```python
from build123d import *

# Parameters (mm, degrees)
BOSS_EXTRUDE1_DEPTH = 4
CUT_EXTRUDE1_REACH  = 42.756
SKETCH2_R           = 2
SKETCH2_R_2         = 2.75
SKETCH2_R_3         = 15
SKETCH4_W           = 4
SKETCH4_H           = 51.1
BOSS_EXTRUDE2_DEPTH = 37
CUT_EXTRUDE2_REACH  = 75.219
SKETCH5_R           = 2.75
CHAMFER2_SIZE       = 30


with BuildPart() as part:
    # Sketch1 → Boss-Extrude1 (new body)
    with BuildSketch(Plane.XY):
        Polygon((-31.5, 21.15), (-31.5, -21.15), (-31.5, -25.55), (31.5, -25.55), (31.5, -21.15), (31.5, 21.15), (31.5, 25.55), (-31.5, 25.55), align=None)
    extrude(amount=BOSS_EXTRUDE1_DEPTH)

    # Sketch2 → Cut-Extrude1 (cut, up to next)
    with BuildSketch(Plane.XY.offset(4), mode=Mode.PRIVATE) as cut_extrude1_sk1:
        with Locations((-5.2, 15.55)):
            Circle(SKETCH2_R)
    cut_extrude1_tool1 = extrude(cut_extrude1_sk1.sketch, amount=-CUT_EXTRUDE1_REACH, mode=Mode.PRIVATE) & part.part
    # Sketch2 → Cut-Extrude1 (cut, up to next)
    with BuildSketch(Plane.XY.offset(4), mode=Mode.PRIVATE) as cut_extrude1_sk2:
        with Locations((25.9, 15.55)):
            Circle(SKETCH2_R)
    cut_extrude1_tool2 = extrude(cut_extrude1_sk2.sketch, amount=-CUT_EXTRUDE1_REACH, mode=Mode.PRIVATE) & part.part
    # Sketch2 → Cut-Extrude1 (cut, up to next)
    with BuildSketch(Plane.XY.offset(4), mode=Mode.PRIVATE) as cut_extrude1_sk3:
        with Locations((25.9, -15.55)):
            Circle(SKETCH2_R)
    cut_extrude1_tool3 = extrude(cut_extrude1_sk3.sketch, amount=-CUT_EXTRUDE1_REACH, mode=Mode.PRIVATE) & part.part
    # Sketch2 → Cut-Extrude1 (cut, up to next)
    with BuildSketch(Plane.XY.offset(4), mode=Mode.PRIVATE) as cut_extrude1_sk4:
        with Locations((-5.2, -15.55)):
            Circle(SKETCH2_R)
    cut_extrude1_tool4 = extrude(cut_extrude1_sk4.sketch, amount=-CUT_EXTRUDE1_REACH, mode=Mode.PRIVATE) & part.part
    # Sketch2 → Cut-Extrude1 (cut, up to next)
    with BuildSketch(Plane.XY.offset(4), mode=Mode.PRIVATE) as cut_extrude1_sk5:
        with Locations((-21.5, 15.55)):
            Circle(SKETCH2_R_2)
    cut_extrude1_tool5 = extrude(cut_extrude1_sk5.sketch, amount=-CUT_EXTRUDE1_REACH, mode=Mode.PRIVATE) & part.part
    # Sketch2 → Cut-Extrude1 (cut, up to next)
    with BuildSketch(Plane.XY.offset(4), mode=Mode.PRIVATE) as cut_extrude1_sk6:
        with Locations((-21.5, -15.55)):
            Circle(SKETCH2_R_2)
    cut_extrude1_tool6 = extrude(cut_extrude1_sk6.sketch, amount=-CUT_EXTRUDE1_REACH, mode=Mode.PRIVATE) & part.part
    # Sketch2 → Cut-Extrude1 (cut, up to next)
    with BuildSketch(Plane.XY.offset(4), mode=Mode.PRIVATE) as cut_extrude1_sk7:
        with Locations((10.35, 0)):
            Circle(SKETCH2_R_3)
    cut_extrude1_tool7 = extrude(cut_extrude1_sk7.sketch, amount=-CUT_EXTRUDE1_REACH, mode=Mode.PRIVATE) & part.part
    add(cut_extrude1_tool1.solids().sort_by_distance((-5.2, 15.55, 4))[0], mode=Mode.SUBTRACT)
    add(cut_extrude1_tool2.solids().sort_by_distance((25.9, 15.55, 4))[0], mode=Mode.SUBTRACT)
    add(cut_extrude1_tool3.solids().sort_by_distance((25.9, -15.55, 4))[0], mode=Mode.SUBTRACT)
    add(cut_extrude1_tool4.solids().sort_by_distance((-5.2, -15.55, 4))[0], mode=Mode.SUBTRACT)
    add(cut_extrude1_tool5.solids().sort_by_distance((-21.5, 15.55, 4))[0], mode=Mode.SUBTRACT)
    add(cut_extrude1_tool6.solids().sort_by_distance((-21.5, -15.55, 4))[0], mode=Mode.SUBTRACT)
    add(cut_extrude1_tool7.solids().sort_by_distance((10.35, 0, 4))[0], mode=Mode.SUBTRACT)

    # Sketch4 → Boss-Extrude2 (add)
    with BuildSketch(Plane(origin=(31.5, 0, 0), x_dir=(0, 0, -1), z_dir=(1, 0, 0))):
        with Locations((-2, 0)):
            Rectangle(SKETCH4_W, SKETCH4_H)
    extrude(amount=BOSS_EXTRUDE2_DEPTH)

    # Sketch5 → Cut-Extrude2 (cut, up to next)
    with BuildSketch(Plane.XY.offset(4), mode=Mode.PRIVATE) as cut_extrude2_sk1:
        with Locations((58.5, -15.55)):
            Circle(SKETCH5_R)
    cut_extrude2_tool1 = extrude(cut_extrude2_sk1.sketch, amount=-CUT_EXTRUDE2_REACH, mode=Mode.PRIVATE) & part.part
    add(cut_extrude2_tool1.solids().sort_by_distance((58.5, -15.55, 4))[0], mode=Mode.SUBTRACT)

    # Chamfer2
    chamfer2_edges = [part.edges().sort_by_distance(p)[0] for p in [
        (68.5, 25.55, 2),
    ]]
    chamfer(chamfer2_edges, length=CHAMFER2_SIZE)


solid = part.part
```
Verification items for the finished model (mm, model axes). Round coordinates to 2 decimals unless told otherwise and drop trailing zeros. Order: outer loops, then holes, each group sorted by start corner. A loop starts at its lowest first (then second) coordinate and runs counter-clockwise, first axis right, second up. Notation, with made-up numbers: (63.25, 6.5) -> (101.25, 6.5) arc R12 ccw to (101.25, 13.5) -> close; hole circle Ø5 at (54, 42.5). An arc over 180 degrees is marked (long way). Put each result on its own line as item: value. Start each with the question number.
(1) Draft check along X on faces 1 (the face through (-24.247, 15.671, 2.028)), 2 (the face through (3, 25.55, 2)), 3 (the face through (68.5, -15, 2)). Enter one of: +X half, -X half, draft (parallel to the pull), parting line (faces both ways), or undercut.
(2) Section check C-C (x = -21.5). Enter the section's corners in (y, z).
(3) Depth check by flat-ended pin: pin 1 Ø1.5 at (y, z) = (9.5, 0.5) entering from +X. Enter the tip coordinate at first touch or a pass-through.
(4) Section check B-B (y = 0). Enter the section's corners in (x, z).
(5) Material ranges on line 1 along Y through (x, z) = (-5.2, 1.7); line 2 along Y through (x, z) = (10.35, 2.35); line 3 along X through (y, z) = (-16.5, 2.45), recorded low to high.
(6) Section check A-A (x = 10.35). Enter the section's corners in (y, z), then the cut area to 3 significant figures.
(7) Section check D-D (z = 1.85). State how many separate pieces and enclosed holes the cut face has, then the cut area to 3 significant figures.
Completed:
1. face 1: undercut
1. face 2: draft
1. face 3: +X half
2. outline: (-25.55, 0) -> (-18.3, 0) -> (-18.3, 4) -> (-25.55, 4) -> close; (-12.8, 0) -> (12.8, 0) -> (12.8, 4) -> (-12.8, 4) -> close; (18.3, 0) -> (25.55, 0) -> (25.55, 4) -> (18.3, 4) -> close
3. pin 1: stops at x = 55.3
4. outline: (-31.5, 0) -> (-4.65, 0) -> (-4.65, 4) -> (-31.5, 4) -> close; (25.35, 0) -> (64.05, 0) -> (64.05, 4) -> (25.35, 4) -> close
5. line 1: y = -25.55 to -17.55, -13.55 to 13.55, 17.55 to 25.55
5. line 2: y = -25.55 to -15, 15 to 25.55
5. line 3: x = -31.5 to -24.08, -18.92 to -6.96, -3.44 to 24.14, 27.66 to 55.92, 61.08 to 68.5
6. outline: (-25.55, 0) -> (-15, 0) -> (-15, 4) -> (-25.55, 4) -> close; (15, 0) -> (25.55, 0) -> (25.55, 4) -> (15, 4) -> close
6. area: 84.4 mm2
7. separate pieces: 1
7. enclosed holes: 8
7. area: 3,830 mm2
